For this review, take the finished solid that the model builds, in its own axes (mm). A direction names the side the tool comes from. Coordinates: 2 decimals unless noted, no trailing zeros. Order: outer loops, then holes, each group sorted by start corner. A loop starts at its lowest first (then second) coordinate and runs counter-clockwise, first axis right, second up. Notation, with made-up numbers: (55.5, 62.5) -> (107.5, 62.5) arc R22 cw to (107.5, 87.5) -> close; hole circle Ø10 at (-8, 26.5). An arc over 180 degrees is marked (long way). Answer as a JSON object with one key per item and string values. Group by question number.
1) Draft analysis for pull direction Y (two halves, no side actions). For faces 1 (the cylindrical face through (-1.972, 3.105, 1.615)), 2 (the flat face through (-2, 0, 0)), 3 (the flat face through (-3.014, 0.76, 1.293)), 4 (the flat face through (14, 0, 0)), state which applies: +Y half, -Y half, draft (parallel to the pull), parting line (faces both ways), or undercut.
2) For pin 1 (1 mm diameter, centred on x = -1.5, z = 1, fed in from +Y); pin 2 (0.9 mm diameter, centred on y = -0.5, z = -0.5, fed in from -X), all flat-tipped, find the tip position at first contact; note any pin that passes through.
3) Wall thickness on L1, parallel to X at y = 1.75, z = 1; L2, parallel to Y at x = -3, z = -1.25; L3, parallel to X at y = 0, z = 0.5: over which ranges is each line inside the solid? List them lowest first.
4) Machinability: for faces 5 (the flat face through (-3, 1.5, 0)), 6 (the flat face through (0, 2, 1)), 7 (the flat face through (-4, 2, 0)), which of the approach directions +Z, -Z, +X, -X, +Y, -Y give a long, thin tool a straight path to every point of the face, cutting with its end or side? Answer none if there is none.
5) Add section A-A, the plane x = -2.5. Write out the cut boundary in (y, z).
6) Add section C-C, the plane y = -1.25. Write out the cut boundary in (x, z).
7) Add section B-B, the plane z = 0. Write out the cut boundary in (x, y), then the cut area to 3 significant figures.
8) Add section D-D, the plane x = 11.75. Write out the cut boundary in (y, z), then the cut area to 3 significant figures.
from build123d import *

# Parameters (mm, degrees)
SOCKET_DEPTH = 2


with BuildPart() as part:
    # Screw Sketch → Screw (revolve)
    with BuildSketch(Plane.XY, mode=Mode.PRIVATE) as screw_sk:
        Polygon((-4, 0), (-4, 3.5), (0, 3.5), (0, 1.65), (14, 1.65), (14, 0), align=None)
    revolve(screw_sk.sketch.rotate(Axis((-1000, 0, 0), (1, 0, 0)), 90), axis=Axis((-1000, 0, 0), (1, 0, 0)))

    # Socket Sketch → Socket (cut)
    with BuildSketch(Plane(origin=(-4, 0, 0), x_dir=(0, 0, -1), z_dir=(1, 0, 0))):
        Polygon((1.732050808, 0), (0.866025404, 1.5), (-0.866025404, 1.5), (-1.732050808, 0), (-0.866025404, -1.5), (0.866025404, -1.5), align=None)
    extrude(amount=SOCKET_DEPTH, mode=Mode.SUBTRACT)


solid = part.part
Output values:
{
 "1": {"face 1": "parting line", "face 2": "undercut", "face 3": "undercut", "face 4": "draft"},
 "2": {"pin 1": "stops at y = 3.46", "pin 2": "stops at x = -2"},
 "3": {"L1": "x = -4 to 0", "L2": "y = -3.27 to -0.83, 0.83 to 3.27", "L3": "x = -2 to 14"},
 "4": {"face 5": "-X", "face 6": "+X", "face 7": "+Z, -Z, -X, +Y, -Y"},
 "5": {"outline": "circle Ø7 at (0, 0); hole (-1.5, -0.87) -> (0, -1.73) -> (1.5, -0.87) -> (1.5, 0.87) -> (0, 1.73) -> (-1.5, 0.87) -> close"},
 "6": {"outline": "(-4, -3.27) -> (0, -3.27) -> (0, -1.08) -> (14, -1.08) -> (14, 1.08) -> (0, 1.08) -> (0, 3.27) -> (-4, 3.27) -> (-4, 1.01) -> (-2, 1.01) -> (-2, -1.01) -> (-4, -1.01) -> close"},
 "7": {"outline": "(-4, -3.5) -> (0, -3.5) -> (0, -1.65) -> (14, -1.65) -> (14, 1.65) -> (0, 1.65) -> (0, 3.5) -> (-4, 3.5) -> (-4, 1.5) -> (-2, 1.5) -> (-2, -1.5) -> (-4, -1.5) -> close", "area": "68.2 mm²"},
 "8": {"outline": "circle Ø3.3 at (0, 0)", "area": "8.55 mm²"}
}
